Model file for the job. Use its own axes, mm. A direction names the side the tool comes from. Coordinates: 2 decimals unless noted, no trailing zeros. Write each loop counter-clockwise with the first axis right and the second up, starting at its lowest first coordinate (ties: lowest second). Pieces come first, ordered by that corner, then holes. Notation, with made-up numbers: (74.5, -27) -> (98.5, -27) arc R20 ccw to (98.5, -11) -> close; hole circle Ø1 at (70.5, -33.5). An arc over 180 degrees is marked (long way). Write item = value, one per line. Start each with the question number.
from build123d import *

# Parameters (mm, degrees)
SKETCH2_W                 = 50
SKETCH2_H                 = 30
SKETCH2_R                 = 3.35
BOSS_EXTRUDE1_DEPTH       = 15
F_8_32_TAPPED_HOLE1_D     = 3.4544
F_8_32_TAPPED_HOLE1_DEPTH = 5
F_8_32_TAPPED_HOLE1_TIP   = 1.037806461
FILLET1_R                 = 3
FILLET2_R                 = 3
FILLET3_R                 = 3
FILLET4_R                 = 3


with BuildPart() as part:
    # Sketch2 → Boss-Extrude1 (new body)
    with BuildSketch(Plane.XY):
        Rectangle(SKETCH2_W, SKETCH2_H)
        with Locations((20, 10)):
            Circle(SKETCH2_R, mode=Mode.SUBTRACT)
        with Locations((-20, 10)):
            Circle(SKETCH2_R, mode=Mode.SUBTRACT)
        with Locations((-20, -10)):
            Circle(SKETCH2_R, mode=Mode.SUBTRACT)
        with Locations((20, -10)):
            Circle(SKETCH2_R, mode=Mode.SUBTRACT)
    extrude(amount=BOSS_EXTRUDE1_DEPTH)

    # #8-32 Tapped Hole1
    with Locations(Plane(origin=(0, 15, 7.5), x_dir=(0, 0, 1), z_dir=(0, 1, 0))):
        with Locations((0, 0)):
            Hole(F_8_32_TAPPED_HOLE1_D / 2, depth=F_8_32_TAPPED_HOLE1_DEPTH)
            with Locations((0, 0, -(F_8_32_TAPPED_HOLE1_DEPTH + F_8_32_TAPPED_HOLE1_TIP / 2))):  # 118° drill point
                Cone(0, F_8_32_TAPPED_HOLE1_D / 2, F_8_32_TAPPED_HOLE1_TIP, mode=Mode.SUBTRACT)

    # Fillet1
    fillet1_edges = [part.edges().sort_by_distance(p)[0] for p in [
        (25, 15, 7.5),
    ]]
    fillet(fillet1_edges, radius=FILLET1_R)

    # Fillet2
    fillet2_edges = [part.edges().sort_by_distance(p)[0] for p in [
        (-25, 15, 7.5),
    ]]
    fillet(fillet2_edges, radius=FILLET2_R)

    # Fillet3
    fillet3_edges = [part.edges().sort_by_distance(p)[0] for p in [
        (25, -15, 7.5),
    ]]
    fillet(fillet3_edges, radius=FILLET3_R)

    # Fillet4
    fillet4_edges = [part.edges().sort_by_distance(p)[0] for p in [
        (-25, -15, 7.5),
    ]]
    fillet(fillet4_edges, radius=FILLET4_R)


solid = part.part
(1) Drop flat-ended pins along their axis: pin 1 Ø10.5 at (x, y) = (20, -10) entering from +Z; pin 2 Ø5.5 at (x, y) = (-20, -10) entering from -Z (3 decimals). Give the stop position or say it passes through.
(2) 3-axis set-ups, long thin cutter, end or side, ignore diameter. For faces 1 (the face through (0.076, 12.465, 9.226)), 2 (the face through (17.342, -12.038, 7.395)): which of +Z, -Z, +X, -X, +Y, -Y reach the whole face in a straight line?
(3) Saw through at B-B (y = 12.5). Give the cut face in (x, z), then the cut area to 3 significant figures.
(4) Saw through at C-C (z = 1.5). Give the cut face in (x, y).
(5) Saw through at D-D (y = -10). Give the cut face in (x, z).
(6) Saw through at A-A (x = -20). Give the cut face in (y, z).
(7) Drill centre lines: line 1 along Y through (x, z) = (20, 11); line 2 along Y through (x, z) = (-17.5, 10); line 3 along X through (y, z) = (-11.5, 5.75). Where is each one in solid material? Low to high.
(8) Mould opens along Z. For faces 3 (the face through (-24.1, -14.14, 7.6)), 4 (the face through (0.013, 9.142, 7.2)), 5 (the face through (0, 0, 0)) say: released by +Z, released by -Z, zero draft, split by the parting line, or undercut.
Returned:
q1.pin_1 = 15
q1.pin_2 = through
q2.face_1 = +Y
q2.face_2 = +Z, -Z
q3.outline = (-24.96, 0) -> (-22.23, 0) -> (-22.23, 15) -> (-24.96, 15) -> close; (-17.77, 0) -> (17.77, 0) -> (17.77, 15) -> (-17.77, 15) -> close; (22.23, 0) -> (24.96, 0) -> (24.96, 15) -> (22.23, 15) -> close; hole circle Ø3.45 at (0, 7.5)
q3.area = 606 mm2
q4.outline = (-25, -12) arc R3 ccw to (-22, -15) -> (22, -15) arc R3 ccw to (25, -12) -> (25, 12) arc R3 ccw to (22, 15) -> (-22, 15) arc R3 ccw to (-25, 12) -> close; hole circle Ø6.7 at (-20, -10); hole circle Ø6.7 at (-20, 10); hole circle Ø6.7 at (20, -10); hole circle Ø6.7 at (20, 10)
q5.outline = (-25, 0) -> (-23.35, 0) -> (-23.35, 15) -> (-25, 15) -> close; (-16.65, 0) -> (16.65, 0) -> (16.65, 15) -> (-16.65, 15) -> close; (23.35, 0) -> (25, 0) -> (25, 15) -> (23.35, 15) -> close
q6.outline = (-15, 0) -> (-13.35, 0) -> (-13.35, 15) -> (-15, 15) -> close; (-6.65, 0) -> (6.65, 0) -> (6.65, 15) -> (-6.65, 15) -> close; (13.35, 0) -> (15, 0) -> (15, 15) -> (13.35, 15) -> close
q7.line_1 = -15 to -13.35, -6.65 to 6.65, 13.35 to 15
q7.line_2 = -15 to -12.23, -7.77 to 7.77, 12.23 to 15
q7.line_3 = -25 to -23, -17 to 17, 23 to 25
q8.face_3 = zero draft
q8.face_4 = undercut
q8.face_5 = released by -Z
